```python
from build123d import *

# Parameters (mm, degrees)
F0_W     = 120
F0_H     = 40.5
F0_W_2   = 115
F0_H_2   = 30.5
F1_DEPTH = 4
F2_W     = 40.5
F2_H     = 11.0000007078
F2_R     = 1.5
F2_H_2   = 4
F3_DEPTH = 5
F4_R     = 1.5
F5_DEPTH = 4
F4_W     = 27.5345724076
F4_H     = 3
F4_H_2   = 0.2320672698
F4_H_3   = 7
F4_H_4   = 3.7679327302
F6_DEPTH = 4.001


with BuildPart() as f1:
    # F0 (on Top) → F1 (new body)
    with BuildSketch(Plane.XY):
        Rectangle(F0_W, F0_H)
        Rectangle(F0_W_2, F0_H_2, mode=Mode.SUBTRACT)
    extrude(amount=F1_DEPTH)

    # F2 (on face) → F3 (join)
    with BuildSketch(Plane(origin=(-60, 0, 0), x_dir=(0, -1, 0), z_dir=(-1, 0, 0))):
        with Locations((0, -5.5000003539)):
            Rectangle(F2_W, F2_H)
        with Locations((-6.25, -2)):
            Circle(F2_R, mode=Mode.SUBTRACT)
        with Locations((0, 2)):
            Rectangle(F2_W, F2_H_2)
    extrude(amount=-F3_DEPTH)

    # F4 (on face) → F5 (join)
    with BuildSketch(Plane(origin=(57.5, 0, 0), x_dir=(0, -1, 0), z_dir=(-1, 0, 0))):
        Polygon((25, 0.2320672698), (25, 20.6540079332), (13.8721717522, 20.6540079332), (13.8721717522, 13.6540079332), (-13.8721717522, 13.6540079332), (-13.8721717522, 20.6540079332), (-25, 20.6540079332), (-25, 0.2320672698), (-15.25, 0.2320672698), (-15.25, 4), (-13.7672862038, 4), (-13.7672862038, 7), (13.7672862038, 7), (13.7672862038, 4), (15.25, 4), (15.25, 0.2320672698), align=None)
        with Locations((-20.25, 10.5)):
            Circle(F4_R, mode=Mode.SUBTRACT)
        with Locations((20.25, 10.5)):
            Circle(F4_R, mode=Mode.SUBTRACT)
    extrude(amount=-F5_DEPTH)

    # F4 (on face) → F6 (cut, through all)
    with BuildSketch(Plane(origin=(57.5, 0, 0), x_dir=(0, -1, 0), z_dir=(-1, 0, 0))):
        with Locations((0, 5.5)):
            Rectangle(F4_W, F4_H)
        with Locations((0, 0.1160336349)):
            Rectangle(F4_W, F4_H_2)
        with Locations((0, -3.5)):
            Rectangle(F4_W, F4_H_3)
        with Locations((0, 2.1160336349)):
            Rectangle(F4_W, F4_H_4)
    extrude(amount=-F6_DEPTH, mode=Mode.SUBTRACT)


solid = f1.part
```
Geometry check sheet. Reference: the model listing, model coordinates, mm. A direction names the side the tool comes from. Round coordinates to 2 decimals unless told otherwise and drop trailing zeros. Loops run counter-clockwise (first coordinate to the right, second up) from the corner with the lowest first, then second, coordinate; pieces in that order, holes last. Notation, with made-up numbers: (56, 24) -> (102, 24) arc R21 ccw to (102, 57) -> close; hole circle Ø7 at (34, -7.75). An arc over 180 degrees is marked (long way). Use a Markdown table: item, result.
(1) Sectioned sample at B-B (y = -9). Enter the section's corners in (x, z), then the cut area to 3 significant figures.
Calculated:
| item | result |
|---|---|
| outline | (-60, -11) -> (-55, -11) -> (-55, 4) -> (-60, 4) -> close; (57.5, 7) -> (61.5, 7) -> (61.5, 13.65) -> (57.5, 13.65) -> close |
| area | 102 mm² |
(2) Mould release check, pull along X, two halves, no side actions. Record for faces 4 (the flat face through (61.5, 0, 11)), 5 (the flat face through (0, -15.25, 2)), 6 (the flat face through (59, 0, 13.654)): released by +X, released by -X, zero draft, split by the parting line, or undercut.
Calculated:
| item | result |
|---|---|
| face 4 | released by +X |
| face 5 | undercut |
| face 6 | zero draft |
(3) Go/stop test with flat-tipped pins: P1, Ø3, axis at x = -20.5, y = 16, coming from the -Z side; P2, Ø1.2, axis at x = 16.5, z = 2, coming from the -Y side; P3, Ø4.5, axis at y = 1, z = -7, coming from the +X side; P4, Ø16.5, axis at y = -10, z = 6.5, coming from the -X side. Record where each tip stops, or that it passes through.
Calculated:
| item | result |
|---|---|
| P1 | z = 0 |
| P2 | y = -20.25 |
| P3 | x = -55 |
| P4 | x = -60 |
(4) Set-up check for faces 1 (the flat face through (2, 18, 0)), 2 (the cylindrical face through (-57.54, 7.36, -0.99)), 3 (the flat face through (59, -13.767, 3)): record each of +Z, -Z, +X, -X, +Y, -Y from which the full face is reachable in a straight line by a thin tool's end or side.
Calculated:
| item | result |
|---|---|
| face 1 | -Z, +X, +Y, -Y |
| face 2 | +X, -X |
| face 3 | -Z, +X |
(5) Sectioned sample at A-A (z = 10.5). Enter the section's corners in (x, y).
Calculated:
| item | result |
|---|---|
| outline | (57.5, -25) -> (61.5, -25) -> (61.5, -21.75) -> (57.5, -21.75) -> close; (57.5, -18.75) -> (61.5, -18.75) -> (61.5, 18.75) -> (57.5, 18.75) -> close; (57.5, 21.75) -> (61.5, 21.75) -> (61.5, 25) -> (57.5, 25) -> close |
(6) Sectioned sample at D-D (y = 6.25). Enter the section's corners in (x, z), then the cut area to 3 significant figures.
Calculated:
| item | result |
|---|---|
| outline | (-60, -11) -> (-55, -11) -> (-55, -3.5) -> (-60, -3.5) -> close; (-60, -0.5) -> (-55, -0.5) -> (-55, 4) -> (-60, 4) -> close; (57.5, 7) -> (61.5, 7) -> (61.5, 13.65) -> (57.5, 13.65) -> close |
| area | 86.6 mm² |
(7) Scan lines: probe 1 along Z at (x, y) = (-57.6, 6.25); probe 2 along Y at (x, z) = (59, 10); probe 3 along X at (y, z) = (23, 0.5). Record each from-to range of solid material in increasing order.
Calculated:
| item | result |
|---|---|
| probe 1 | -11 to -3.5, -0.5 to 4 |
| probe 2 | -25 to -21.66, -18.84 to 18.84, 21.66 to 25 |
| probe 3 | 57.5 to 61.5 |
(8) Sectioned sample at C-C (x = -6). Enter the section's corners in (y, z).
Calculated:
| item | result |
|---|---|
| outline | (-20.25, 0) -> (-15.25, 0) -> (-15.25, 4) -> (-20.25, 4) -> close; (15.25, 0) -> (20.25, 0) -> (20.25, 4) -> (15.25, 4) -> close |
